Autodesk Inventor part; units mm, degrees
ref_plane "YZ Plane" through (0, 0, 0) normal (1, 0, 0) x (0, 1, 0)
ref_plane "XZ Plane" through (0, 0, 0) normal (0, 1, 0) x (-1, 0, 0)
ref_plane "XY Plane" through (0, 0, 0) normal (0, 0, 1) x (1, 0, 0)
sketch "スケッチ1" plane through (0, 0, 0) normal (0, 0, 1) x (1, 0, 0)
  line L0 (-101.5, 47.999998) -> (108.5, 47.999998)
  circle A0 centre (111.885049, -19.000002) radius 4
  circle A1 centre (171.880735, -19.719469) radius 4
  circle A2 centre (111.885049, -19.000002) radius 7
  circle A3 centre (171.880735, -19.719469) radius 7
  line L1 (171.880735, -19.719469) -> (111.885049, -19.000002) construction
  line L2 (171.964673, -12.719973) -> (111.968987, -12.000505)
  line L3 (111.801111, -25.999499) -> (171.796797, -26.718966)
  arc A4 (171.796797, -26.718966) -> (171.964673, -12.719973) centre (171.880735, -19.719469) ccw
  arc A5 (111.968987, -12.000505) -> (111.801111, -25.999499) centre (111.885049, -19.000002) ccw
  line L4 (173.796111, -12.986614) -> (250.19065, -34.719469)
  circle A6 centre (241.981901, -63.574563) radius 30
  line L5 (268.180017, -78.191633) -> (221.951227, -41.241357)
  line L6 (221.951227, -41.241357) -> (169.96536, -26.452325)
  line L7 (271.981901, -113.136134) -> (271.981901, -54.819928)
  line L8 (111.885049, -19.000002) -> (111.885049, 40.999998) construction
  line L9 (118.885049, -19.000002) -> (118.885049, 40.999998)
  line L10 (104.885049, 40.999998) -> (104.885049, -19.000002)
  arc A7 (104.885049, -19.000002) -> (118.885049, -19.000002) centre (111.885049, -19.000002) ccw
  arc A8 (118.885049, 40.999998) -> (104.885049, 40.999998) centre (111.885049, 40.999998) ccw
  circle A9 centre (29.431848, 47.237971) radius 30
  line L11 (113.319325, 34.148513) -> (35.578744, 17.874462)
  line L12 (-0.558472, 47.999998) -> (57.548937, 36.777124)
  line L13 (57.548937, 36.777124) -> (110.450773, 47.851484)
  circle A10 centre (113.5, -20.000002) radius 68
  line L14 (321.963533, -82.955067) -> (60.270532, 100.284345)
  line L15 (259.189194, -39.000002) -> (111.885049, -19.000002)
  arc A11 (93.592427, -27.104845) -> (135.370976, -5.924402) centre (95.060351, 21.794105) ccw
  arc A12 (135.370976, -5.924402) -> (135.847591, -3.671647) centre (132.898992, -4.224609) ccw
  arc A13 (135.847591, -3.671647) -> (83.183341, 18.55647) centre (102.157897, -9.989602) ccw
  line L16 (111.885049, -19.000002) -> (112.689188, 40.994609) construction
  line L17 (118.88442, -19.093818) -> (119.688559, 40.900793)
  line L18 (105.689816, 41.088425) -> (104.885678, -18.906186)
  arc A14 (104.885678, -18.906186) -> (118.88442, -19.093818) centre (111.885049, -19.000002) ccw
  arc A15 (119.688559, 40.900793) -> (105.689816, 41.088425) centre (112.689188, 40.994609) ccw
  line L19 (164.994898, 47.999998) -> (164.994898, 25.999998)
  line L20 (164.994898, 25.999998) -> (327.494898, -102.000002)
  circle A16 centre (116.292557, -40.000002) radius 68
  circle A17 centre (-98.885049, -0.000002) radius 67.5
  line L21 (321.363327, -8.500986) -> (-152.668056, 78.49822)
  line L22 (104.889695, -3) -> (104.889695, 0)
  line L23 (104.889695, -3) -> (72.06562, -3)
  line L24 (72.06562, 0) -> (104.889695, 0)
  circle A18 centre (83.376901, -17.5) radius 13.85
  line L25 (178.77046, -28.957215) -> (174.212284, -32.858886)
  line L26 (174.212284, -32.858886) -> (164.880735, -30.20423)
  line L27 (164.880735, -30.20423) -> (164.880735, -19.719469)
  line L28 (169.96536, -26.452325) -> (168.597236, -31.261507)
  line L29 (168.597236, -31.261507) -> (164.880735, -26.636029)
  line L30 (178.880232, -19.803408) -> (178.654717, -38.608867)
  line L31 (165.012544, -21.071485) -> (158.172386, 13.676274)
  circle A19 centre (171.880735, -19.719469) radius 7.5
  point P0 (0, 0)
  point P1 (0, 0)
  point P2 (141.882892, -19.359736)
  point P3 (111.885049, 10.999998)
  point P4 (105.885049, -0.000002)
  point P5 (105.885049, -0.000002)
  point P6 (23.732778, -42.728965)
  point P7 (112.287118, 10.997304)
  point P8 (169.272284, -12.687685)
  point P9 (163.348193, -12.616644)
  point P10 (164.492485, -18.429603)
  point P11 (172.555184, -27.189082)
  point P12 (178.847945, -22.495796)
  point P13 (170.863298, -26.707772)
  dimension "d0" = 8
  dimension "d1" = 8
  dimension "d2" = 3
  dimension "d3" = 3
  dimension "d4" = 60
  dimension "d5" = 14
  dimension "d6" = 14
  dimension "d7" = 60
  dimension "d8" = 14
  dimension "d9" = 60
  dimension "d10" = 14
  dimension "d11" = 6
  dimension "d12" = 35
  dimension "d13" = 13.271
  dimension "d14" = 14
  dimension "d15" = 20
  dimension "d16" = 15
  dimension "d17" = 22
  dimension "d18" = 150
  dimension "d19" = 162.5
  dimension "d20" = 0
  dimension "d21" = 136
  dimension "d22" = 136
  dimension "d23" = 135
  dimension "d24" = 38.2272
  dimension "d25" = 18
  dimension "d26" = 5
  dimension "d27" = 6
  dimension "d28" = 101.823
  dimension "d29" = 101.823
  dimension "d30" = 0.5
extrude "押し出し1" add sketch "スケッチ1" against normal blind 5 contours A10 L15 A16 L6 | L6 L30 L15 A10 | A16 L15 A6 L6 | L6 L15 L30 | L15 L30 A19 L4 A16 A10 | A10 A16 L15 | A6 L15 L20 L5 | A16 A10 L4 L20 A6 L15 | L6 A19 L30 L15 | A16 L4 A10 | A6 L20 L15 | L6 L3 A3 L30 A19 | L30 A3 L4 A19 | L20 L4 A6 | A6 L15 L20 | L15 A6 L20 | A3 | A1
hole "穴1" at (105.885049, -0.000002, 0) at (113.5, -20.000002, 0) at (23.732778, -42.728965, 0) at (116.292557, -40.000002, 0) at (-98.885049, -0.000002, 0) at (171.880735, -19.719469, 0) direction (0, 0, -1) diameter 8.05 depth 12 tip angle 118
sketch "スケッチ2" plane through (0, 0, 0) normal (0, 0, 1) x (1, 0, 0)
  circle A0 centre (171.880735, -19.719469) radius 4.025
  arc A1 (268.180017, -78.191633) -> (250.19065, -34.719469) centre (241.981901, -63.574563) ccw
  line L0 (268.180017, -78.191633) -> (221.951227, -41.241357)
  line L1 (221.951227, -41.241357) -> (170.863298, -26.707772)
  line L2 (170.863298, -26.707772) -> (171.796797, -26.718966)
  arc A2 (173.796111, -12.986614) -> (171.796797, -26.718966) centre (171.880735, -19.719469) ccw
  line L3 (173.796111, -12.986614) -> (250.19065, -34.719469)
  circle A3 centre (171.880735, -19.719469) radius 7
  circle A4 centre (171.880735, -19.719469) radius 8.5
  point P0 (0, 0)
  point P1 (178.433917, -14.305986)
  point P2 (174.603168, -27.771696)
  dimension "d40" = 1.5
extrude "押し出し2" add sketch "スケッチ2" against normal blind 5 contours L3 A2 L2 L1 A4
sketch "スケッチ3" plane through (0, 0, 0) normal (0, 0, 1) x (1, 0, 0)
  circle A0 centre (171.880735, -19.719469) radius 4.025
  arc A1 (268.180017, -78.191633) -> (250.19065, -34.719469) centre (241.981901, -63.574563) ccw
  line L0 (268.180017, -78.191633) -> (221.951227, -41.241357)
  line L1 (221.951227, -41.241357) -> (174.603168, -27.771696)
  arc A2 (178.433917, -14.305986) -> (174.603168, -27.771696) centre (171.880735, -19.719469) ccw
  line L2 (178.433917, -14.305986) -> (250.19065, -34.719469)
  circle A3 centre (171.880735, -19.719469) radius 6
  point P0 (0, 0)
  dimension "d43" = 12
extrude "押し出し3" cut sketch "スケッチ3" against normal blind 1 contours A3
equation "\"d9\" = d7"
equation "\"d29\" = d28"
properties part number "後ろウィング先端"
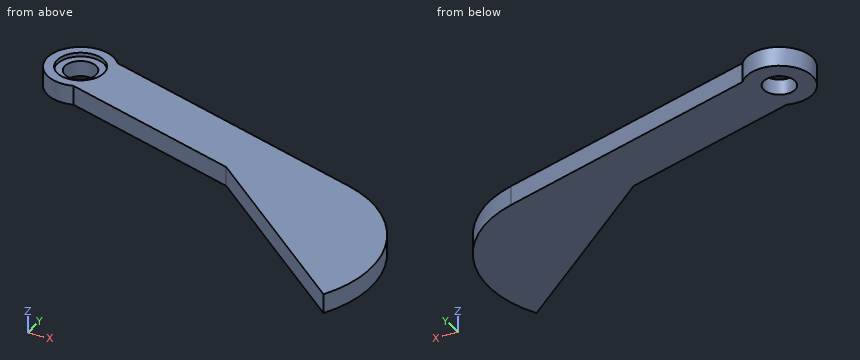
Source: CAD feature listing. Evaluate the final solid. Frame: model axes, mm. Coordinates: 2 decimals unless noted, no trailing zeros. Loops run counter-clockwise (first coordinate to the right, second up) from the corner with the lowest first, then second, coordinate; pieces in that order, holes last. Notation, with made-up numbers: M -15,-32 L 4,-32 A13 ccw 4,-20 Z; hole C -11.5,77 d2. An arc over 180 degrees is marked long. Use a Markdown table: item, result. Add a question column.
Q1. Section query C-C, the plane y = -44. Return loops of the section in (x, z), and give its area (3 significant figures).
Q2. Section query A-A, the plane z = -2.4. Return loops of the section in (x, y) (3 decimals), and give its area (3 significant figures).
Q3. First-contact query: pin 1 (5 mm diameter, centred on x = 241, y = -28, fed in from -Z); pin 2 (11 mm diameter, centred on x = 171.88, y = -19.72, fed in from +Z); pin 3 (1 mm diameter, centred on x = 251.5, z = -0.5, fed in from -Y); pin 4 (3 mm diameter, centred on x = 235.5, z = -3, fed in from -Y). Flat tips, straight axial feed; report the tip coordinate or a pass-through.
Q4. Section query B-B, the plane x = 242. Return loops of the section in (y, z).
Q5. Material intervals for L1, parallel to Z at x = 175.5, y = -24; L2, parallel to Y at x = 180.5, z = -4.4; L3, parallel to X at y = -52, z = -1.1, sorted ascending.
Result:
| question | item | result |
|---|---|---|
| 1 | outline | M 225.4,-5 L 264.72,-5 L 264.72,0 L 225.4,0 Z |
| 1 | area | 197 mm2 |
| 2 | outline | M 174.603,-27.772 L 221.951,-41.241 L 268.18,-78.192 A30 ccw 250.191,-34.719 L 178.434,-14.306 A8.5 ccw long Z; hole C 171.881,-19.719 d8.05 |
| 2 | area | 2,050 mm2 |
| 3 | pin 1 | passes through |
| 3 | pin 2 | stops at z = -1 |
| 3 | pin 3 | stops at y = -65.26 |
| 3 | pin 4 | stops at y = -53.27 |
| 4 | outline | M -57.27,-5 L -32.39,-5 L -32.39,0 L -57.27,0 Z |
| 5 | L1 | z = -5 to -1 |
| 5 | L2 | y = -29.45 to -14.89 |
| 5 | L3 | x = 235.41 to 269.66 |
